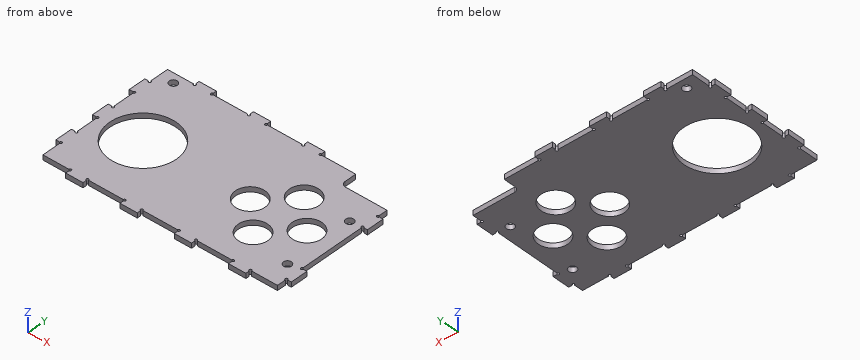
```python
from build123d import *

# Parameters (mm, degrees)
SKETCH_5_W          = 95
SKETCH_5_H          = 56
EXTRUDE_1_DEPTH     = 2
SKETCH_3_R          = 6
CUT_EXTRUDE_2_DEPTH = 106.577578112
SKETCH_4_R          = 13.5
CUT_EXTRUDE_3_DEPTH = 106.577578112
SKETCH_6_W          = 20
SKETCH_6_H          = 9
CUT_EXTRUDE_4_DEPTH = 106.577578112
FILLET_2_R          = 2
SKETCH_8_R          = 1.6
CUT_EXTRUDE_6_DEPTH = 106.577578112
SKETCH_10_W         = 7
SKETCH_10_H         = 2
EXTRUDE_2_DEPTH     = 2
SKETCH_11_R         = 0.5
CUT_EXTRUDE_8_DEPTH = 107.628443672
SKETCH_12_W         = 2
SKETCH_12_H         = 7
EXTRUDE_3_DEPTH     = 2
SKETCH_13_W         = 2
SKETCH_13_H         = 7
EXTRUDE_4_DEPTH     = 2
SKETCH_14_R         = 0.5
CUT_EXTRUDE_9_DEPTH = 109.326474142


with BuildPart() as part:
    # 草图5 → 凸台-拉伸1 (new body)
    with BuildSketch(Plane.XY):
        with Locations((42.75, 26.75)):
            Rectangle(SKETCH_5_W, SKETCH_5_H)
    extrude(amount=EXTRUDE_1_DEPTH)

    # 草图3 → 切除-拉伸2 (cut, through all)
    with BuildSketch(Plane.XY):
        with Locations((67.5, 36)):
            Circle(SKETCH_3_R)
        with Locations((56, 24.5)):
            Circle(SKETCH_3_R)
        with Locations((67.5, 13)):
            Circle(SKETCH_3_R)
        with Locations((79, 24.5)):
            Circle(SKETCH_3_R)
    extrude(amount=CUT_EXTRUDE_2_DEPTH, mode=Mode.SUBTRACT)

    # 草图4 → 切除-拉伸3 (cut, through all)
    with BuildSketch(Plane.XY):
        with Locations((13, 24)):
            Circle(SKETCH_4_R)
    extrude(amount=CUT_EXTRUDE_3_DEPTH, mode=Mode.SUBTRACT)

    # 草图6 → 切除-拉伸4 (cut, through all)
    with BuildSketch(Plane.XY):
        with Locations((81.5, 52.5)):
            Rectangle(SKETCH_6_W, SKETCH_6_H)
    extrude(amount=CUT_EXTRUDE_4_DEPTH, mode=Mode.SUBTRACT)

    # 圆角2
    fillet_2_edges = [part.edges().sort_by_distance(p)[0] for p in [
        (71.5, 48, 1),
    ]]
    fillet(fillet_2_edges, radius=FILLET_2_R)

    # 草图8 → 切除-拉伸6 (cut, through all)
    with BuildSketch(Plane(origin=(0, 0, 0), x_dir=(-1, 0, 0), z_dir=(0, 0, -1))):
        with Locations((-85.5, 36.5)):
            Circle(SKETCH_8_R)
        with Locations((-85.5, 8.5)):
            Circle(SKETCH_8_R)
        with Locations((-1, 51)):
            Circle(SKETCH_8_R)
    extrude(amount=-CUT_EXTRUDE_6_DEPTH, mode=Mode.SUBTRACT)

    # 草图10 → 凸台-拉伸2 (add)
    with BuildSketch(Plane(origin=(0, 0, 0), x_dir=(-1, 0, 0), z_dir=(0, 0, -1))):
        with Locations((-9.75, 55.75)):
            Rectangle(SKETCH_10_W, SKETCH_10_H)
        with Locations((-31.75, 55.75)):
            Rectangle(SKETCH_10_W, SKETCH_10_H)
        with Locations((-53.75, 55.75)):
            Rectangle(SKETCH_10_W, SKETCH_10_H)
        with Locations((-75.75, -2.25)):
            Rectangle(SKETCH_10_W, SKETCH_10_H)
        with Locations((-53.75, -2.25)):
            Rectangle(SKETCH_10_W, SKETCH_10_H)
        with Locations((-31.75, -2.25)):
            Rectangle(SKETCH_10_W, SKETCH_10_H)
        with Locations((-9.75, -2.25)):
            Rectangle(SKETCH_10_W, SKETCH_10_H)
    extrude(amount=-EXTRUDE_2_DEPTH)

    # 草图11 → 切除-拉伸8 (cut, through all)
    with BuildSketch(Plane(origin=(0, 0, 0), x_dir=(-1, 0, 0), z_dir=(0, 0, -1))):
        with Locations((-57.25, 54.75)):
            Circle(SKETCH_11_R)
        with Locations((-50.25, 54.75)):
            Circle(SKETCH_11_R)
        with Locations((-35.25, 54.75)):
            Circle(SKETCH_11_R)
        with Locations((-28.25, 54.75)):
            Circle(SKETCH_11_R)
        with Locations((-13.25, 54.75)):
            Circle(SKETCH_11_R)
        with Locations((-6.25, 54.75)):
            Circle(SKETCH_11_R)
        with Locations((-79.25, -1.25)):
            Circle(SKETCH_11_R)
        with Locations((-72.25, -1.25)):
            Circle(SKETCH_11_R)
        with Locations((-57.25, -1.25)):
            Circle(SKETCH_11_R)
        with Locations((-50.25, -1.25)):
            Circle(SKETCH_11_R)
        with Locations((-35.25, -1.25)):
            Circle(SKETCH_11_R)
        with Locations((-28.25, -1.25)):
            Circle(SKETCH_11_R)
        with Locations((-13.25, -1.25)):
            Circle(SKETCH_11_R)
        with Locations((-6.25, -1.25)):
            Circle(SKETCH_11_R)
    extrude(amount=-CUT_EXTRUDE_8_DEPTH, mode=Mode.SUBTRACT)

    # 草图12 → 凸台-拉伸3 (add)
    with BuildSketch(Plane.XY.offset(2)):
        with Locations((91.25, 40.5)):
            Rectangle(SKETCH_12_W, SKETCH_12_H)
        with Locations((91.25, 6.25)):
            Rectangle(SKETCH_12_W, SKETCH_12_H)
    extrude(amount=-EXTRUDE_3_DEPTH)

    # 草图13 → 凸台-拉伸4 (add)
    with BuildSketch(Plane.XY.offset(2)):
        with Locations((-5.75, 10.25)):
            Rectangle(SKETCH_13_W, SKETCH_13_H)
        with Locations((-5.75, 26.75)):
            Rectangle(SKETCH_13_W, SKETCH_13_H)
        with Locations((-5.75, 43.25)):
            Rectangle(SKETCH_13_W, SKETCH_13_H)
    extrude(amount=-EXTRUDE_4_DEPTH)

    # 草图14 → 切除-拉伸9 (cut, through all)
    with BuildSketch(Plane.XY.offset(2)):
        with Locations((-4.75, 46.75)):
            Circle(SKETCH_14_R)
        with Locations((-4.75, 39.75)):
            Circle(SKETCH_14_R)
        with Locations((-4.75, 30.25)):
            Circle(SKETCH_14_R)
        with Locations((-4.75, 23.25)):
            Circle(SKETCH_14_R)
        with Locations((-4.75, 13.75)):
            Circle(SKETCH_14_R)
        with Locations((-4.75, 6.75)):
            Circle(SKETCH_14_R)
        with Locations((90.25, 44)):
            Circle(SKETCH_14_R)
        with Locations((90.25, 37)):
            Circle(SKETCH_14_R)
        with Locations((90.25, 9.75)):
            Circle(SKETCH_14_R)
        with Locations((90.25, 2.75)):
            Circle(SKETCH_14_R)
    extrude(amount=-CUT_EXTRUDE_9_DEPTH, mode=Mode.SUBTRACT)


solid = part.part
```
Can you work these out from the model? Positions are in its coordinate system, mm. Give positions to 0.01 mm unless a question says otherwise; leave off trailing zeros. Loops run counter-clockwise (first coordinate to the right, second up) from the corner with the lowest first, then second, coordinate; pieces in that order, holes last. Notation, with made-up numbers: M -7,69.5 L 50,69.5 A22 ccw 50,84.5 Z; hole C 29,6.5 d2. An arc over 180 degrees is marked long. Use CSV: the item, a comma, the result in double quotes. Start each with the question number.
1. For P1, Ø0.8, axis at y = -2, z = 1, coming from the -X side; P2, Ø0.8, axis at y = -2.5, z = 1, coming from the +X side; P3, Ø8, axis at x = 12.5, y = 18.5, coming from the +Z side; P4, Ø1, axis at x = 19.5, z = 0.5, coming from the -Y side, each with a flat end and sliding along its axis, tell me the tip position at first contact or that it passes through.
2. Imagine slicing it at A-A, the plane x = 69. Write out the boundary of the cut face in (y, z), plus the area to 3 significant figures.
3. Imagine slicing it at D-D, the plane y = 16. Write out the boundary of the cut face in (x, z).
4. If I drill on L1, parallel to Y at x = 85.5, z = 0.3; L2, parallel to X at y = 32, z = 0.15; L3, parallel to X at y = 29, z = 1.5, over which ranges is the centre line in solid material (lowest first)?
5. Imagine slicing it at C-C, the plane x = 19. Write out the boundary of the cut face in (y, z).
6. Imagine slicing it at B-B, the plane y = 28. Write out the boundary of the cut face in (x, z).
Response values:
1,P1,"x = 6.25"
1,P2,"x = 79.25"
1,P3,"through"
1,P4,"y = -1.25"
2,outline,"M -1.25,0 L 7.19,0 L 7.19,2 L -1.25,2 Z; M 18.81,0 L 30.19,0 L 30.19,2 L 18.81,2 Z; M 41.81,0 L 54.75,0 L 54.75,2 L 41.81,2 Z"
2,area,"65.5 mm^2"
3,outline,"M -4.75,0 L 2.13,0 L 2.13,2 L -4.75,2 Z; M 23.87,0 L 62.3,0 L 62.3,2 L 23.87,2 Z; M 72.7,0 L 90.25,0 L 90.25,2 L 72.7,2 Z"
4,L1,"-1.25 to 6.9, 10.1 to 34.9, 38.1 to 48"
4,L2,"-4.75 to 2.13, 23.87 to 63.03, 71.97 to 90.25"
4,L3,"-6.75 to 0.46, 25.54 to 52.03, 59.97 to 75.03, 82.97 to 90.25"
5,outline,"M -1.25,0 L 11.91,0 L 11.91,2 L -1.25,2 Z; M 36.09,0 L 54.75,0 L 54.75,2 L 36.09,2 Z"
6,outline,"M -6.75,0 L 0.11,0 L 0.11,2 L -6.75,2 Z; M 25.89,0 L 51.13,0 L 51.13,2 L 25.89,2 Z; M 60.87,0 L 74.13,0 L 74.13,2 L 60.87,2 Z; M 83.87,0 L 90.25,0 L 90.25,2 L 83.87,2 Z"
